Geometry check sheet. Reference: the model listing, model coordinates, mm. A direction names the side the tool comes from. Coordinates: 2 decimals unless noted, no trailing zeros. Write each loop counter-clockwise with the first axis right and the second up, starting at its lowest first coordinate (ties: lowest second). Pieces come first, ordered by that corner, then holes. Notation, with made-up numbers: (71.25, 13) -> (111.25, 13) arc R12 cw to (111.25, 26) -> close; hole circle Ø6 at (-13.75, 49.25). An arc over 180 degrees is marked (long way). One line per question, with ' | ' between items.
```python
from build123d import *

# Parameters (mm, degrees)
SKETCH2_R           = 7.5
BOSS_EXTRUDE1_DEPTH = 5
CUT_EXTRUDE1_DEPTH  = 4


with BuildPart() as part:
    # Sketch2 → Boss-Extrude1 (new, symmetric)
    with BuildSketch(Plane(origin=(0, 0, 0), x_dir=(0, 0, -1), z_dir=(1, 0, 0))):
        with BuildLine():
            Line((50, 0), (-50, 0))
            Line((-50, 0), (-20, 180))
            ThreePointArc((-20, 180), (0, 200), (20, 180))
            Line((20, 180), (50, 0))
        make_face()
        with Locations((0, 180)):
            Circle(SKETCH2_R, mode=Mode.SUBTRACT)
    extrude(amount=BOSS_EXTRUDE1_DEPTH, both=True)

    # Sketch3 → Cut-Extrude1 (cut)
    with BuildSketch(Plane.ZY.offset(5)):
        Polygon((0, 33), (-35, 33), (-35, 39), (35, 39), (35, 33), align=None)
    extrude(amount=-CUT_EXTRUDE1_DEPTH, mode=Mode.SUBTRACT)


solid = part.part
```
(1) Cross-section at D-D (y = 19.5). Record the cut outline in (x, z), plus the area to 3 significant figures.
Answers below:
outline: (-5, -46.75) -> (5, -46.75) -> (5, 46.75) -> (-5, 46.75) -> close | area: 935 mm²
(2) Draft check along Z on faces 1 (the face through (0.07, 88.74, 35.21)), 2 (the face through (0, 0, -1)), 3 (the face through (-3, 33, 0)). Enter one of: pulls with the +Z half, pulls with the -Z half, needs draft (parallel to the pull), parting line crosses it, or undercut.
Answers below:
face 1: pulls with the +Z half | face 2: needs draft | face 3: undercut
(3) Material ranges on line 1 (Y direction, x = 2, z = 0); line 2 (Z direction, x = -1.5, y = 178); line 3 (Z direction, x = -2, y = 185), recorded low to high.
Answers below:
line 1: y = 0 to 172.5, 187.5 to 200 | line 2: z = -20.33 to -7.23, 7.23 to 20.33 | line 3: z = -19.36 to -5.59, 5.59 to 19.36
(4) Cross-section at B-B (z = 0). Record the cut outline in (x, y).
Answers below:
outline: (-5, 0) -> (5, 0) -> (5, 172.5) -> (-5, 172.5) -> (-5, 39) -> (-1, 39) -> (-1, 33) -> (-5, 33) -> close; (-5, 187.5) -> (5, 187.5) -> (5, 200) -> (-5, 200) -> close
(5) Cross-section at A-A (x = 2). Record the cut outline in (y, z), plus the area to 3 significant figures.
Answers below:
outline: (0, -50) -> (180, -20) arc R20 ccw to (180, 20) -> (0, 50) -> close; hole circle Ø15 at (180, 0) | area: 13,100 mm²
(6) Tool access check on faces 4 (the face through (-3, 39, 0)), 5 (the face through (-0.07, 187.436, 0.976)). Record the directions out of +Z, -Z, +X, -X, +Y, -Y that give a thin tool (end or side, any length) a straight path to the whole face; none if there is none.
Answers below:
face 4: -X | face 5: +X, -X
(7) Depth check by flat-ended pin: P1, Ø1, axis at x = -2, y = 171.5, coming from the -Z side; P2, Ø2, axis at x = -2.5, y = 37.5, coming from the +Z side; P3, Ø2, axis at x = -2.5, y = 36.5, coming from the -Z side. Enter the tip coordinate at first touch or a pass-through.
Answers below:
P1: stops at z = -21.5 | P2: stops at z = 43.92 | P3: stops at z = -44.08
(8) Cross-section at C-C (z = -32). Record the cut outline in (x, y), plus the area to 3 significant figures.
Answers below:
outline: (-5, 0) -> (5, 0) -> (5, 108) -> (-5, 108) -> (-5, 39) -> (-1, 39) -> (-1, 33) -> (-5, 33) -> close | area: 1,060 mm²
